```python
from build123d import *

# Parameters (mm, degrees)
F0_W     = 60
F0_H     = 30
F1_DEPTH = 25
F2_W     = 54
F2_H     = 3.5
F3_DEPTH = 30.001
F4_W     = 54
F4_H     = 24
F5_DEPTH = 15
F6_W     = 3
F6_H     = 4
F7_DEPTH = 3
F8_R     = 1.177089
F9_DEPTH = 25.001


with BuildPart() as f1:
    # F0 (on Top) → F1 (new body)
    with BuildSketch(Plane.XY):
        with Locations((-0.009455, -0.203341)):
            Rectangle(F0_W, F0_H)
    extrude(amount=F1_DEPTH)

    # F2 (on face) → F3 (cut, through all)
    with BuildSketch(Plane.XZ.offset(15.203341)):
        with Locations((-0.009455, 4.75)):
            Rectangle(F2_W, F2_H)
    extrude(amount=-F3_DEPTH, mode=Mode.SUBTRACT)

    # F4 (on face) → F5 (cut)
    with BuildSketch(Plane.XY.offset(25)):
        with Locations((-0.009455, -0.203341)):
            Rectangle(F4_W, F4_H)
    extrude(amount=-F5_DEPTH, mode=Mode.SUBTRACT)

    # F6 (on face) → F7 (cut)
    with BuildSketch(Plane.XY.offset(25)):
        with Locations((28.490545, -0.203341)):
            Rectangle(F6_W, F6_H)
    extrude(amount=-F7_DEPTH, mode=Mode.SUBTRACT)

    # F8 (on face) → F9 (cut, through all)
    with BuildSketch(Plane.XY.offset(25)):
        with Locations((25.990545, 13.288478)):
            Circle(F8_R)
        with Locations((-26.009455, 13.296659)):
            Circle(F8_R)
        with Locations((-26.009455, -13.703341)):
            Circle(F8_R)
        with Locations((25.990545, -13.703341)):
            Circle(F8_R)
    extrude(amount=-F9_DEPTH, mode=Mode.SUBTRACT)


solid = f1.part
```
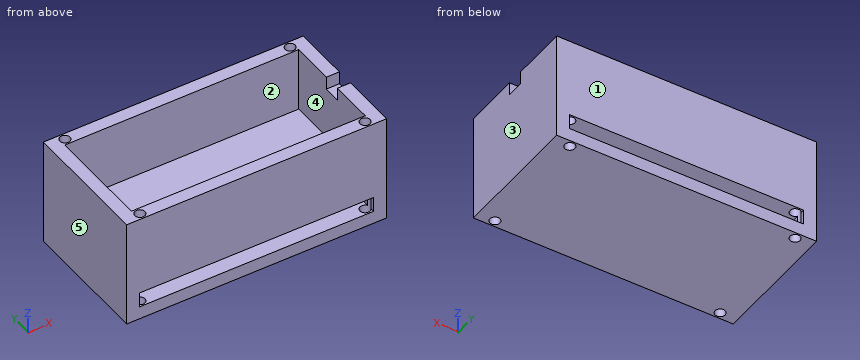
Geometry check sheet. Reference: the model listing, model coordinates, mm. Face numbers are marked on the shaded views. A direction names the side the tool comes from. Round coordinates to 2 decimals unless told otherwise and drop trailing zeros. Order: outer loops, then holes, each group sorted by start corner. A loop starts at its lowest first (then second) coordinate and runs counter-clockwise, first axis right, second up. Notation, with made-up numbers: (20, -35) - (71, -35) arc R20 ccw to (71, -18) - close; hole circle Ø10 at (48, 10). An arc over 180 degrees is marked (long way). Use a Markdown table: item, result. Add a question column.
(1) Material ranges on line 1 along Z through (x, y) = (-23, 2.5); line 2 along X through (y, z) = (-12, 10.5); line 3 along Y through (x, z) = (20.5, 14.5), recorded low to high. Write a range as [from, to].
(2) Depth check by flat-ended pin: pin 1 (6 mm diameter, centred on x = 3, y = 7.5, fed in from +Z); pin 2 (1.4 mm diameter, centred on x = 25.99, y = -13.7, fed in from -Z); pin 3 (2.5 mm diameter, centred on x = 28, y = 0.5, fed in from +Z). Enter the tip coordinate at first touch or a pass-through.
(3) Sectioned sample at B-B, the plane y = 6. Enter the section's corners in (x, z).
(4) Sectioned sample at A-A, the plane x = -12. Enter the section's corners in (y, z).
(5) Release check for a two-part mould opening along X. For the marked faces 1, 2 and 3 record: pulls with the +X half, pulls with the -X half, needs draft (parallel to the pull), parting line crosses it, or undercut.
(6) Tool access check on the marked faces 4 and 5. Record the directions out of +Z, -Z, +X, -X, +Y, -Y that give a thin tool (end or side, any length) a straight path to the whole face; none if there is none.
(7) Sectioned sample at C-C, the plane z = 20.25. Enter the section's corners in (x, y).
Answers below:
| question | item | result |
|---|---|---|
| 1 | line 1 | [0, 3], [6.5, 10] |
| 1 | line 2 | [-30.01, -27.01], [26.99, 29.99] |
| 1 | line 3 | [-15.2, -12.2], [11.8, 14.8] |
| 2 | pin 1 | z = 10 |
| 2 | pin 2 | through |
| 2 | pin 3 | z = 22 |
| 3 | outline | (-30.01, 0) - (29.99, 0) - (29.99, 25) - (26.99, 25) - (26.99, 10) - (-27.01, 10) - (-27.01, 25) - (-30.01, 25) - close; hole (-27.01, 3) - (26.99, 3) - (26.99, 6.5) - (-27.01, 6.5) - close |
| 4 | outline | (-15.2, 0) - (14.8, 0) - (14.8, 3) - (-15.2, 3) - close; (-15.2, 6.5) - (14.8, 6.5) - (14.8, 25) - (11.8, 25) - (11.8, 10) - (-12.2, 10) - (-12.2, 25) - (-15.2, 25) - close |
| 5 | face 1 | needs draft |
| 5 | face 2 | undercut |
| 5 | face 3 | pulls with the +X half |
| 6 | face 4 | +Z |
| 6 | face 5 | +Z, -Z, -X, +Y, -Y |
| 7 | outline | (-30.01, -15.2) - (29.99, -15.2) - (29.99, 14.8) - (-30.01, 14.8) - close; hole circle Ø2.35 at (-26.01, -13.7); hole circle Ø2.35 at (-26.01, 13.3); hole (-27.01, -12.2) - (26.99, -12.2) - (26.99, 11.8) - (-27.01, 11.8) - close; hole circle Ø2.35 at (25.99, -13.7); hole circle Ø2.35 at (25.99, 13.29) |
